Design review of the part built by this model. Coordinates are the model's own, in mm. Face numbers are marked on the shaded views. A direction names the side the tool comes from. Give positions to 0.01 mm unless a question says otherwise; leave off trailing zeros. Loops run counter-clockwise (first coordinate to the right, second up) from the corner with the lowest first, then second, coordinate; pieces in that order, holes last. Notation, with made-up numbers: (85.5, 2.25) -> (114.5, 2.25) arc R24 ccw to (114.5, 19.25) -> close; hole circle Ø10 at (82, 22). An arc over 180 degrees is marked (long way). Answer in a Markdown table with one row per item. Add a question column.
(1) For line 1 (X direction, y = 2.45, z = -22.5); line 2 (X direction, y = -1.75, z = -7.5); line 3 (Z direction, x = 40.75, y = 2.05), list the stretches that pass through material, from the lowest coordinate up.
(2) Consider section A-A on y = -0.5. Write out the cut boundary in (x, z).
(3) Consider section B-B on z = -22.5. Write out the cut boundary in (x, y), then the cut area to 3 significant figures.
(4) For pin 1 (2.5 mm diameter, centred on x = 3.75, z = -22.5, fed in from +Y); pin 2 (1 mm diameter, centred on x = 18, z = -22, fed in from -Y); pin 3 (5 mm diameter, centred on x = 7, y = -7.5, fed in from -Z); pin 4 (2.5 mm diameter, centred on x = 19, y = 2, fed in from +Z), all flat-tipped, find the tip position at first contact; note any pin that passes through.
(5) Consider section C-C on z = -11. Write out the cut boundary in (x, y).
(6) For the marked faces 1, 2 and 3, list the 3-axis set-ups (+Z, -Z, +X, -X, +Y, -Y) from which the entire face can be reached by the end or side of a thin tool; tool diameter is ignored.
(7) Draft analysis for pull direction X (two halves, no side actions). For the marked faces 4, 5 and 6, state which applies: +X half, -X half, draft (parallel to the pull), parting line (faces both ways), or undercut.
(8) Consider section D-D on x = 3.75. Write out the cut boundary in (y, z).
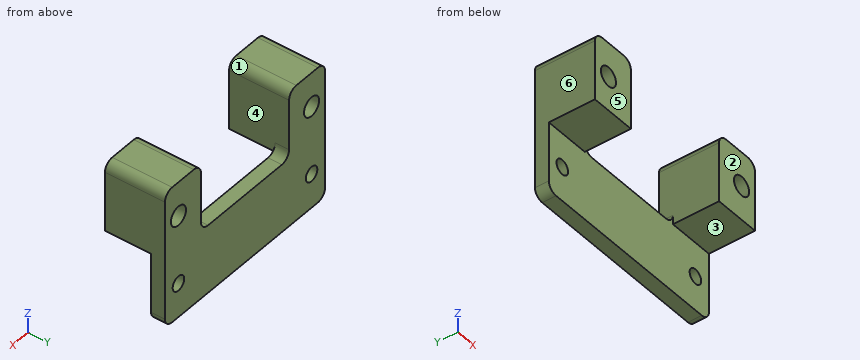
from build123d import *

# Parameters (mm, degrees)
SKETCH_1_W          = 44.5
SKETCH_1_H          = 30
EXTRUDE_1_DEPTH     = 3
SKETCH_2_W          = 10
SKETCH_2_H          = 15
EXTRUDE_2_DEPTH     = 10
SKETCH_3_R          = 2.1
SKETCH_3_R_2        = 1.6
CUT_EXTRUDE_1_DEPTH = 45
SKETCH_4_W          = 24.5
SKETCH_4_H          = 15
CUT_EXTRUDE_2_DEPTH = 10
FILLET_2_R          = 2


with BuildPart() as part:
    # ｽｹｯﾁ1 → ﾎﾞｽ - 押し出し1 (new body)
    with BuildSketch(Plane(origin=(0, 0, 0), x_dir=(1, 0, 0), z_dir=(0, 1, 0))):
        with Locations((22.25, 15)):
            Rectangle(SKETCH_1_W, SKETCH_1_H)
    extrude(amount=EXTRUDE_1_DEPTH)

    # ｽｹｯﾁ2 → ﾎﾞｽ - 押し出し2 (add)
    with BuildSketch(Plane(origin=(0, 0, 0), x_dir=(-1, 0, 0), z_dir=(0, -1, 0))):
        with Locations((-5, 7.5)):
            Rectangle(SKETCH_2_W, SKETCH_2_H)
        with Locations((-39.5, 7.5)):
            Rectangle(SKETCH_2_W, SKETCH_2_H)
    extrude(amount=EXTRUDE_2_DEPTH)

    # ｽｹｯﾁ3 → ｶｯﾄ - 押し出し1 (cut)
    with BuildSketch(Plane(origin=(0, 3, 0), x_dir=(1, 0, 0), z_dir=(0, 1, 0))):
        with Locations((3.75, 7.5)):
            Circle(SKETCH_3_R)
        with Locations((40.75, 7.5)):
            Circle(SKETCH_3_R)
        with Locations((40.75, 22.5)):
            Circle(SKETCH_3_R_2)
        with Locations((3.75, 22.5)):
            Circle(SKETCH_3_R_2)
    extrude(amount=-CUT_EXTRUDE_1_DEPTH, mode=Mode.SUBTRACT)

    # ｽｹｯﾁ4 → ｶｯﾄ - 押し出し2 (cut)
    with BuildSketch(Plane(origin=(0, 0, 0), x_dir=(-1, 0, 0), z_dir=(0, -1, 0))):
        with Locations((-22.25, 7.5)):
            Rectangle(SKETCH_4_W, SKETCH_4_H)
    extrude(amount=-CUT_EXTRUDE_2_DEPTH, mode=Mode.SUBTRACT)

    # ﾌｨﾚｯﾄ2
    fillet_2_edges = [part.edges().sort_by_distance(p)[0] for p in [
        (10, -3.5, 0),
        (34.5, -3.5, 0),
        (10, 1.5, -15),
        (34.5, 1.5, -15),
        (0, 1.5, -30),
        (44.5, 1.5, -30),
        (44.5, -3.5, 0),
        (0, -3.5, 0),
    ]]
    fillet(fillet_2_edges, radius=FILLET_2_R)


solid = part.part
Values follow:
| question | item | result |
|---|---|---|
| 1 | line 1 | 0 to 2.15, 5.35 to 39.15, 42.35 to 44.5 |
| 1 | line 2 | 0 to 1.65, 5.85 to 10, 34.5 to 38.65, 42.85 to 44.5 |
| 1 | line 3 | -30 to -24.1, -20.9 to -9.6, -5.4 to 0 |
| 2 | outline | (0, -15) -> (10, -15) -> (10, -2) arc R2 ccw to (8, 0) -> (2, 0) arc R2 ccw to (0, -2) -> close; (34.5, -15) -> (44.5, -15) -> (44.5, -2) arc R2 ccw to (42.5, 0) -> (36.5, 0) arc R2 ccw to (34.5, -2) -> close; hole circle Ø4.2 at (3.75, -7.5); hole circle Ø4.2 at (40.75, -7.5) |
| 3 | outline | (0, 0) -> (2.15, 0) -> (2.15, 3) -> (0, 3) -> close; (5.35, 0) -> (39.15, 0) -> (39.15, 3) -> (5.35, 3) -> close; (42.35, 0) -> (44.5, 0) -> (44.5, 3) -> (42.35, 3) -> close |
| 3 | area | 114 mm2 |
| 4 | pin 1 | through |
| 4 | pin 2 | y = 0 |
| 4 | pin 3 | z = -15 |
| 4 | pin 4 | z = -15 |
| 5 | outline | (0, -10) -> (10, -10) -> (10, 3) -> (0, 3) -> close; (34.5, -10) -> (44.5, -10) -> (44.5, 3) -> (34.5, 3) -> close |
| 6 | face 1 | +Z, +Y, -Y |
| 6 | face 2 | +Z, -Z, +X, -X, -Y |
| 6 | face 3 | -Z, +X, -X, -Y |
| 7 | face 4 | undercut |
| 7 | face 5 | draft |
| 7 | face 6 | -X half |
| 8 | outline | (-10, -15) -> (0, -15) -> (0, -20.9) -> (3, -20.9) -> (3, -9.6) -> (-10, -9.6) -> close; (-10, -5.4) -> (3, -5.4) -> (3, 0) -> (-10, 0) -> close; (0, -30) -> (3, -30) -> (3, -24.1) -> (0, -24.1) -> close |
